Work out the finished part from the listing and answer in its coordinate system (mm). A direction names the side the tool comes from. Round coordinates to 2 decimals unless told otherwise and drop trailing zeros. Order: outer loops, then holes, each group sorted by start corner. A loop starts at its lowest first (then second) coordinate and runs counter-clockwise, first axis right, second up. Notation, with made-up numbers: (41.5, 18.25) - (68.5, 18.25) arc R19 cw to (68.5, 55.25) - close; hole circle Ø7 at (43.25, -7). An arc over 180 degrees is marked (long way). Use one line per item in the form item = value. Start each with the question number.
Q1. Which of the six approach directions +Z, -Z, +X, -X, +Y, -Y give full straight-line access (tool end or side, diameter ignored) to faces 4 (the flat face through (-42.5, 16, 0)), 5 (the flat face through (46, -5, 0)), 6 (the flat face through (-37.5, 13, 0))?
Q2. The part is cut by section A-A on y = -4. Determine the outline of the cut face in (x, z).
Q3. Find the intervals of material crossed by line 1 (X direction, y = 12.5, z = 6); line 2 (X direction, y = -2, z = 2); line 3 (Y direction, x = 24.5, z = -5.75), in increasing order. Write a range as [from, to].
Q4. For a pull along Y with two mould halves and no side action, classify faces 1 (the cylindrical face through (44.62, 4.91, -0.11)), 2 (the flat face through (0, 1, -7.5)), 3 (the flat face through (50, -10, 0)) as +Y half, -Y half, draft (parallel to the pull), parting line (faces both ways), or undercut.
Q5. The part is cut by section D-D on y = 9. Determine the outline of the cut face in (x, z), plus the area to 3 significant figures.
Q6. The part is cut by section C-C on x = -10. Determine the outline of the cut face in (y, z), plus the area to 3 significant figures.
Q7. Given P1, Ø3, axis at x = -31, z = 1, coming from the +Y side; P2, Ø3.5, axis at y = -5, z = -3.5, coming from the -X side; P3, Ø2.5, axis at x = -49.5, z = 3.5, coming from the +Y side, each flat-ended and moving along its own axis, determine where each tip first touches the part or whether it passes through.
Q8. The part is cut by section B-B on z = -4. Determine the outline of the cut face in (x, y).
from build123d import *

# Parameters (mm, degrees)
SKETCH1_W           = 82
SKETCH1_H           = 15
BOSS_EXTRUDE1_DEPTH = 7
SKETCH3_W           = 5
SKETCH3_H           = 15
BOSS_EXTRUDE2_DEPTH = 13
FILLET1_R           = 10
SKETCH4_W           = 5
SKETCH4_H           = 22
BOSS_EXTRUDE3_DEPTH = 15
FILLET2_R           = 6
SKETCH5_W           = 15
SKETCH5_H           = 5
BOSS_EXTRUDE4_DEPTH = 9


with BuildPart() as part:
    # Sketch1 → Boss-Extrude1 (new body)
    with BuildSketch(Plane(origin=(0, 0, 0), x_dir=(1, 0, 0), z_dir=(0, 1, 0))):
        Rectangle(SKETCH1_W, SKETCH1_H)
    extrude(amount=BOSS_EXTRUDE1_DEPTH)

    # Sketch3 → Boss-Extrude2 (add)
    with BuildSketch(Plane(origin=(0, 7, 0), x_dir=(1, 0, 0), z_dir=(0, 1, 0))):
        with Locations((-40, 0)):
            Rectangle(SKETCH3_W, SKETCH3_H)
        with Locations((40, 0)):
            Rectangle(SKETCH3_W, SKETCH3_H)
    extrude(amount=BOSS_EXTRUDE2_DEPTH)

    # Fillet1
    # the kernel refuses this fillet: 10 mm, written as the material it takes off along each edge
    with BuildSketch(Plane(origin=(42.5, 7, -20.669567191), x_dir=(-1, 0, 0), z_dir=(0, 0, 1)), Plane(origin=(-42.5, 7, 20.669567191), x_dir=(1, 0, 0), z_dir=(0, 0, -1))) as fillet1_piece_1:
        with BuildLine():
            CenterArc((10, -5.267826876), FILLET1_R, 148.211669383, 31.788330617)
            Line((0, -5.267826876), (-0.2, -5.267826876))
            Line((-0.2, -5.267826876), (-0.2, 0))
            Line((-0.2, 0), (0, 0.2))
            ThreePointArc((0, 0.2), (0.75, 0.2), (1.33, 0.105356538))
            Line((1.33, 0.105356538), (1.5, 0))
        make_face()
    extrude(amount=41.339134382, mode=Mode.SUBTRACT)

    # Sketch4 → Boss-Extrude3 (add)
    with BuildSketch(Plane(origin=(0, 0, -7.5), x_dir=(-1, 0, 0), z_dir=(0, 0, -1))):
        with Locations((-43.5, -4)):
            Rectangle(SKETCH4_W, SKETCH4_H)
        with Locations((43.5, -4)):
            Rectangle(SKETCH4_W, SKETCH4_H)
    extrude(amount=-BOSS_EXTRUDE3_DEPTH)

    # Fillet2
    # the kernel refuses this fillet: 6 mm, written as the material it takes off along each edge
    with BuildSketch(Plane(origin=(46, 7, -22.290199458), x_dir=(-1, 0, 0), z_dir=(0, 0, 1))) as fillet2_piece_1_section:
        with BuildLine():
            CenterArc((6, 5.916079783), FILLET2_R, 180, 80.405931773)
            Line((0, 5.916079783), (-0.12, 5.916079783))
            Line((-0.12, 5.916079783), (-0.12, 0))
            Line((-0.12, 0), (0, -0.12))
            ThreePointArc((0, -0.12), (2.5, -0.12), (4.98, -0.118321596))
            Line((4.98, -0.118321596), (5, 0))
        make_face()
    fillet2_piece_1 = extrude(amount=44.580398916, mode=Mode.PRIVATE)
    fillet2_piece_1 = fillet2_piece_1 - Plane(origin=(32.5, 12.267826876, 0), x_dir=(-1, 0, 0), z_dir=(0, 0, -1)) * Cylinder(10, 113, mode=Mode.PRIVATE)
    add(fillet2_piece_1, mode=Mode.SUBTRACT)
    with BuildSketch(Plane(origin=(-46, 7, -22.290199458), x_dir=(1, 0, 0), z_dir=(0, 0, 1))) as fillet2_piece_2_section:
        with BuildLine():
            CenterArc((6, -5.916079783), FILLET2_R, 99.594068227, 80.405931773)
            Line((0, -5.916079783), (-0.12, -5.916079783))
            Line((-0.12, -5.916079783), (-0.12, 0))
            Line((-0.12, 0), (0, 0.12))
            ThreePointArc((0, 0.12), (2.5, 0.12), (4.98, 0.118321596))
            Line((4.98, 0.118321596), (5, 0))
        make_face()
    fillet2_piece_2 = extrude(amount=44.580398916, mode=Mode.PRIVATE)
    fillet2_piece_2 = fillet2_piece_2 - Plane(origin=(-32.5, 12.267826876, 0), x_dir=(1, 0, 0), z_dir=(0, 0, 1)) * Cylinder(10, 113, mode=Mode.PRIVATE)
    add(fillet2_piece_2, mode=Mode.SUBTRACT)

    # Sketch5 → Boss-Extrude4 (add)
    with BuildSketch(Plane.ZY.offset(46)):
        with Locations((0, -12.5)):
            Rectangle(SKETCH5_W, SKETCH5_H)
    boss_extrude4 = extrude(amount=BOSS_EXTRUDE4_DEPTH)

    # Mirror1: Boss-Extrude4 across plane
    add(boss_extrude4.mirror(Plane(origin=(0, 0, 0), x_dir=(0, 0, 1), z_dir=(1, 0, 0))))


solid = part.part
Found:
q1.face_4 = +Z, -Z, -X, +Y
q1.face_5 = +Z, -Z, +X, +Y
q1.face_6 = +Z, -Z, +Y
q2.outline = (-46, -7.5) - (-41, -7.5) - (-41, 7.5) - (-46, 7.5) - close; (41, -7.5) - (46, -7.5) - (46, 7.5) - (41, 7.5) - close
q3.line_1 = [-42.5, -37.5], [37.5, 42.5]
q3.line_2 = [-46, -41], [41, 46]
q3.line_3 = [0, 7]
q4.face_1 = undercut
q4.face_2 = draft
q4.face_3 = +Y half
q5.outline = (-41.95, -7.5) - (-37.5, -7.5) - (-37.5, 7.5) - (-41.95, 7.5) - close; (37.5, -7.5) - (41.95, -7.5) - (41.95, 7.5) - (37.5, 7.5) - close
q5.area = 134 mm²
q6.outline = (0, -7.5) - (7, -7.5) - (7, 7.5) - (0, 7.5) - close
q6.area = 105 mm²
q7.P1 = 7
q7.P2 = -46
q7.P3 = -10
q8.outline = (-55, -15) - (-41, -15) - (-41, 0) - (41, 0) - (41, -15) - (55, -15) - (55, -10) - (46, -10) - (46, 1.08) arc R6 ccw to (41, 7) arc R10 ccw to (42.5, 12.27) - (42.5, 20) - (37.5, 20) - (37.5, 7) - (-37.5, 7) - (-37.5, 20) - (-42.5, 20) - (-42.5, 12.27) arc R10 ccw to (-41, 7) arc R6 ccw to (-46, 1.08) - (-46, -10) - (-55, -10) - close
